Work out the finished part from the listing and answer in its coordinate system (mm). Coordinates: 2 decimals unless noted, no trailing zeros. Order: outer loops, then holes, each group sorted by start corner. A loop starts at its lowest first (then second) coordinate and runs counter-clockwise, first axis right, second up. Notation, with made-up numbers: (30, -39.75) - (82, -39.75) arc R24 ccw to (82, -23.75) - close; hole circle Ø11 at (59.25, 42). An arc over 180 degrees is marked (long way). Use CSV: the item, a comma, the result in double quotes. Start each with the question number.
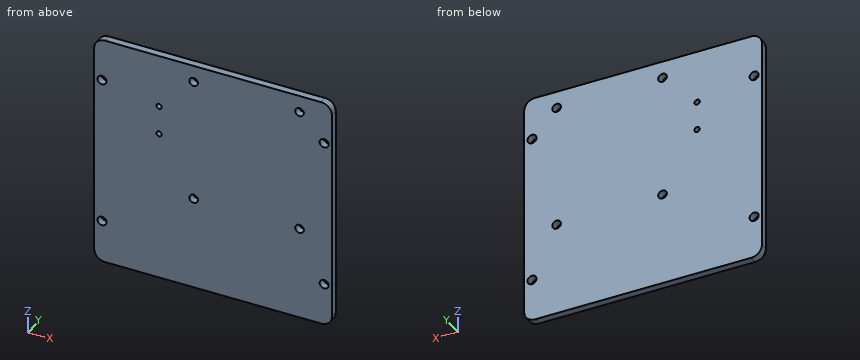
from build123d import *

# Parameters (mm, degrees)
ESQUISSE1_R        = 2.1
BOSS_EXTRU_1_DEPTH = 3.5
CONG_1_R           = 5
ESQUISSE3_R        = 2
TROUS_RPI_DEPTH    = 78.860452092
ESQUISSE5_R        = 1.25
TROUS_ICM_DEPTH    = 78.860452092


with BuildPart() as part:
    # Esquisse1 → Boss.-Extru.1 (new body)
    # profile 1 of 2: a face of its own
    with BuildSketch(Plane(origin=(0, 0, 0), x_dir=(1, 0, 0), z_dir=(0, 1, 0))):
        with BuildLine():
            Line((-55, 31.4), (-55, -55))
            Line((-55, -55), (55, -55))
            Line((55, -55), (55, 55))
            Line((55, 55), (-55, 55))
            Line((-55, 55), (-55, 38.6))
            Line((-55, 38.6), (-51.4, 38.6))
            ThreePointArc((-51.4, 38.6), (-47.8, 35), (-51.4, 31.4))
            Line((-51.4, 31.4), (-55, 31.4))
        make_face()
        with Locations(Location((-51.4, -35, 0), (0, 0, 270))):
            Circle(ESQUISSE1_R, mode=Mode.SUBTRACT)
        with Locations(Location((51.4, -35, 0), (0, 0, 270))):
            Circle(ESQUISSE1_R, mode=Mode.SUBTRACT)
        with Locations(Location((51.4, 35, 0), (0, 0, 270))):
            Circle(ESQUISSE1_R, mode=Mode.SUBTRACT)
    # profile 2 of 2: a face of its own
    with BuildSketch(Plane(origin=(0, 0, 0), x_dir=(1, 0, 0), z_dir=(0, 1, 0))):
        with BuildLine():
            Line((-55, 38.6), (-55, 31.4))
            Line((-55, 31.4), (-51.4, 31.4))
            ThreePointArc((-51.4, 31.4), (-47.8, 35), (-51.4, 38.6))
            Line((-51.4, 38.6), (-55, 38.6))
        make_face()
        with Locations(Location((-51.4, 35, 0), (0, 0, 270))):
            Circle(ESQUISSE1_R, mode=Mode.SUBTRACT)
    extrude(amount=BOSS_EXTRU_1_DEPTH)

    # Congé1
    cong_1_edges = [part.edges().sort_by_distance(p)[0] for p in [
        (55, 1.75, -55),
        (55, 1.75, 55),
        (-55, 1.75, 55),
        (-55, 1.75, -55),
    ]]
    fillet(cong_1_edges, radius=CONG_1_R)

    # Esquisse3 → Trous RPI (cut, through all)
    with BuildSketch(Plane(origin=(0, 3.5, 0), x_dir=(1, 0, 0), z_dir=(0, 1, 0))):
        with Locations(Location((40, 11, 0), (0, 0, 270))):
            Circle(ESQUISSE3_R)
        with Locations(Location((40, -47, 0), (0, 0, 270))):
            Circle(ESQUISSE3_R)
        with Locations(Location((-9, -47, 0), (0, 0, 270))):
            Circle(ESQUISSE3_R)
        with Locations(Location((-9, 11, 0), (0, 0, 270))):
            Circle(ESQUISSE3_R)
    extrude(amount=-TROUS_RPI_DEPTH, mode=Mode.SUBTRACT)

    # Esquisse5 → Trous ICM (cut, through all)
    with BuildSketch(Plane(origin=(0, 0, 0), x_dir=(-1, 0, 0), z_dir=(0, -1, 0))):
        with Locations(Location((25, -30, 0), (0, 0, 90))):
            Circle(ESQUISSE5_R)
        with Locations(Location((25, -16.4, 0), (0, 0, 90))):
            Circle(ESQUISSE5_R)
    extrude(amount=-TROUS_ICM_DEPTH, mode=Mode.SUBTRACT)


solid = part.part
1) Straight lines are drawn through the part: line 1 (X direction, y = 0.85, z = -35); line 2 (X direction, y = 1.25, z = -11); line 3 (Z direction, x = -9.5, y = 2.2). For each, find the intervals that lie inside material, in ascending order. Write a range as [from, to].
2) The part is cut by section B-B on x = 40. Determine the outline of the cut face in (y, z), plus the area to 3 significant figures.
3) The part is cut by section A-A on z = -35. Determine the outline of the cut face in (x, y).
4) A flat-ended cylindrical pin translates along its axis: P1, Ø2, axis at x = -25, z = 16.4, coming from the +Y side. Find the tip coordinate at first contact, or state that the pin passes through.
5) The part is cut by section C-C on z = 16.4. Determine the outline of the cut face in (x, y).
Answer key:
1,line 1,"[-55, -53.5], [-49.3, 49.3], [53.5, 55]"
1,line 2,"[-55, -11], [-7, 38], [42, 55]"
1,line 3,"[-55, -12.94], [-9.06, 45.06], [48.94, 55]"
2,outline,"(0, -55) - (3.5, -55) - (3.5, -13) - (0, -13) - close; (0, -9) - (3.5, -9) - (3.5, 45) - (0, 45) - close; (0, 49) - (3.5, 49) - (3.5, 55) - (0, 55) - close"
2,area,"357 mm^2"
3,outline,"(-55, 0) - (-53.5, 0) - (-53.5, 3.5) - (-55, 3.5) - close; (-49.3, 0) - (49.3, 0) - (49.3, 3.5) - (-49.3, 3.5) - close; (53.5, 0) - (55, 0) - (55, 3.5) - (53.5, 3.5) - close"
4,P1,"through"
5,outline,"(-55, 0) - (-26.25, 0) - (-26.25, 3.5) - (-55, 3.5) - close; (-23.75, 0) - (55, 0) - (55, 3.5) - (-23.75, 3.5) - close"
